Design review of the part built by this model. Coordinates are the model's own, in mm. A direction names the side the tool comes from. Round coordinates to 2 decimals unless told otherwise and drop trailing zeros. Write each loop counter-clockwise with the first axis right and the second up, starting at its lowest first coordinate (ties: lowest second). Pieces come first, ordered by that corner, then holes.
from build123d import *

# Parameters (mm, degrees)
SKETCH1_W                  = 60
SKETCH1_H                  = 40
BOSS_EXTRUDE1_DEPTH        = 4
SKETCH4_R                  = 14.5
CUT_EXTRUDE1_DEPTH         = 4
SKETCH6_R                  = 1.6
CUT_EXTRUDE2_DEPTH         = 4
SKETCH7_W                  = 26
SKETCH7_H                  = 4
BOSS_EXTRUDE3_DEPTH        = 10
SKETCH8_R                  = 1.6
CUT_EXTRUDE3_DEPTH         = 78.162231694
SKETCH9_W                  = 4
SKETCH9_H                  = 4
BOSS_EXTRUDE4_DEPTH        = 12.5
FILLET2_R                  = 4
FILLET3_R                  = 1
SKETCH10_W                 = 6
SKETCH10_H                 = 4
BOSS_EXTRUDE5_DEPTH        = 6
FILLET4_R                  = 6
F_3_2_3_2_DIAMETER_HOLE1_D = 3.2


with BuildPart() as part:
    # Sketch1 → Boss-Extrude1 (new body)
    with BuildSketch(Plane.XY):
        with Locations((30, 20)):
            Rectangle(SKETCH1_W, SKETCH1_H)
    extrude(amount=BOSS_EXTRUDE1_DEPTH)

    # Sketch4 → Cut-Extrude1 (cut)
    with BuildSketch(Plane.XY.offset(4)):
        with Locations((30, 23.5)):
            Circle(SKETCH4_R)
    extrude(amount=-CUT_EXTRUDE1_DEPTH, mode=Mode.SUBTRACT)

    # Sketch6 → Cut-Extrude2 (cut)
    with BuildSketch(Plane.XY.offset(4)):
        with Locations((42, 11.5)):
            Circle(SKETCH6_R)
        with Locations((18, 11.5)):
            Circle(SKETCH6_R)
        with Locations((18, 35.5)):
            Circle(SKETCH6_R)
        with Locations((42, 35.5)):
            Circle(SKETCH6_R)
    extrude(amount=-CUT_EXTRUDE2_DEPTH, mode=Mode.SUBTRACT)

    # Sketch7 → Boss-Extrude3 (add)
    with BuildSketch(Plane.XY.offset(4)):
        with Locations((59.5, 15.6)):
            Rectangle(SKETCH7_W, SKETCH7_H)
    extrude(amount=BOSS_EXTRUDE3_DEPTH)

    # Sketch8 → Cut-Extrude3 (cut, through all)
    with BuildSketch(Plane(origin=(0, 17.6, 0), x_dir=(1, 0, 0), z_dir=(0, 1, 0))):
        with Locations(Location((68.5, -9.75, 0), (0, 0, 270))):
            Circle(SKETCH8_R)
        with Locations(Location((50.5, -9.75, 0), (0, 0, 270))):
            Circle(SKETCH8_R)
    extrude(amount=-CUT_EXTRUDE3_DEPTH, mode=Mode.SUBTRACT)

    # Sketch9 → Boss-Extrude4 (add)
    with BuildSketch(Plane(origin=(60, 0, 0), x_dir=(0, 0, -1), z_dir=(1, 0, 0))):
        with Locations((-2, 15.6)):
            Rectangle(SKETCH9_W, SKETCH9_H)
    extrude(amount=BOSS_EXTRUDE4_DEPTH)

    # Fillet2
    fillet2_edges = [part.edges().sort_by_distance(p)[0] for p in [
        (46.5, 15.6, 14),
        (72.5, 15.6, 14),
        (72.5, 15.6, 0),
    ]]
    fillet(fillet2_edges, radius=FILLET2_R)

    # Fillet3
    fillet3_edges = [part.edges().sort_by_distance(p)[0] for p in [
        (46.5, 15.6, 4),
        (53.25, 13.6, 4),
        (60, 13.6, 2),
    ]]
    fillet(fillet3_edges, radius=FILLET3_R)

    # Sketch10 → Boss-Extrude5 (add)
    with BuildSketch(Plane.XZ):
        with Locations((30, 2)):
            Rectangle(SKETCH10_W, SKETCH10_H)
    extrude(amount=BOSS_EXTRUDE5_DEPTH)

    # Fillet4
    fillet4_edges = [part.edges().sort_by_distance(p)[0] for p in [
        (27, 0, 2),
        (33, 0, 2),
    ]]
    fillet(fillet4_edges, radius=FILLET4_R - 0.0001)  # a hair under: the kernel refuses the full size

    # Ø3.2 (3.2) Diameter Hole1 (through all)
    with Locations(Plane.XY.offset(4)):
        with Locations((30, -3)):
            Hole(F_3_2_3_2_DIAMETER_HOLE1_D / 2)


solid = part.part
1) For P1, Ø4, axis at x = 68.5, z = 9.75, coming from the +Y side; P2, Ø6, axis at y = 31, z = 6.5, coming from the +X side; P3, Ø12, axis at x = 44, y = 4.5, coming from the +Z side; P4, Ø1.9, axis at x = 42, y = 11.5, coming from the +Z side, all flat-tipped, find the tip position at first contact; note any pin that passes through.
2) For line 1 along X through (y, z) = (16.05, 9.75); line 2 along Y through (x, z) = (30, 2.4); line 3 along Y through (x, z) = (18, 1.7), list the stretches that pass through material, from the lowest coordinate up.
3) Add section B-B on x = 30. State the section outline as (y, z) points, and give its area (3 significant figures).
4) For faces 1 (the face through (49, 0, 2)), 2 (the face through (31.6, -2.93, 1.97)), 3 (the face through (10, 0, 2)), list the 3-axis set-ups (+Z, -Z, +X, -X, +Y, -Y) from which the entire face can be reached by the end or side of a thin tool; tool diameter is ignored.
5) Add section C-C on y = 16. State the section outline as (x, z) points.
6) Add section A-A on y = 23.5. State the section outline as (x, z) points.
7) Add section D-D on x = 18. State the section outline as (y, z) points.
8) The part is to be moulded in two halves that separate along X. For faces 4 (the face through (25.196, -1.711, 2.028)), 5 (the face through (34, 6, 0)), 6 (the face through (40.82, 12.58, 2.03)), say which applies: pulls with the +X half, pulls with the -X half, needs draft (parallel to the pull), parting line crosses it, or undercut.
Computed:
1. P1: stops at y = 17.6
1. P2: stops at x = 60
1. P3: stops at z = 4
1. P4: passes through
2. line 1: x = 46.5 to 48.9, 52.1 to 66.9, 70.1 to 72.5
2. line 2: y = -6 to -4.6, -1.4 to 9, 38 to 40
2. line 3: y = 0 to 9.9, 13.1 to 15.36, 31.64 to 33.9, 37.1 to 40
3. outline: (-6, 0) - (-4.6, 0) - (-4.6, 4) - (-6, 4) - close; (-1.4, 0) - (9, 0) - (9, 4) - (-1.4, 4) - close; (38, 0) - (40, 0) - (40, 4) - (38, 4) - close
3. area: 55.2 mm2
4. face 1: +Z, -Z, +X, -Y
4. face 2: +Z, -Z
4. face 3: +Z, -Z, -X, -Y
5. outline: (0, 0) - (17.59, 0) - (17.59, 4) - (0, 4) - close; (42.41, 0) - (68.5, 0) arc R4 ccw to (72.5, 4) - (72.5, 10) arc R4 ccw to (68.5, 14) - (50.5, 14) arc R4 ccw to (46.5, 10) - (46.5, 5) arc R1 cw to (45.5, 4) - (42.41, 4) - close; hole circle Ø3.2 at (50.5, 9.75); hole circle Ø3.2 at (68.5, 9.75)
6. outline: (0, 0) - (15.5, 0) - (15.5, 4) - (0, 4) - close; (44.5, 0) - (60, 0) - (60, 4) - (44.5, 4) - close
7. outline: (0, 0) - (9.9, 0) - (9.9, 4) - (0, 4) - close; (13.1, 0) - (15.36, 0) - (15.36, 4) - (13.1, 4) - close; (31.64, 0) - (33.9, 0) - (33.9, 4) - (31.64, 4) - close; (37.1, 0) - (40, 0) - (40, 4) - (37.1, 4) - close
8. face 4: pulls with the -X half
8. face 5: needs draft
8. face 6: undercut
